from build123d import *

# Parameters (mm, degrees)
BOSS_EXTRUDE1_DEPTH = 3
SKETCH3_W           = 24
SKETCH3_H           = 4
BOSS_EXTRUDE2_DEPTH = 4
SKETCH6_W           = 24
SKETCH6_H           = 4
BOSS_EXTRUDE4_DEPTH = 3
CUT_EXTRUDE1_DEPTH  = 2.3
SKETCH9_W           = 2
SKETCH9_H           = 7
SKETCH9_W_2         = 1.5
BOSS_EXTRUDE5_DEPTH = 3
SKETCH11_W          = 2
SKETCH11_H          = 7
SKETCH11_W_2        = 1.497470588
BOSS_EXTRUDE6_DEPTH = 4
SKETCH10_R          = 1.25
CUT_EXTRUDE2_DEPTH  = 10.5
BOSS_EXTRUDE7_DEPTH = 2


with BuildPart() as part:
    # Sketch1 → Boss-Extrude1 (new body)
    with BuildSketch(Plane(origin=(0, 0, 0), x_dir=(1, 0, 0), z_dir=(0, 1, 0))):
        with BuildLine():
            ThreePointArc((-17.3, 2), (-18.5, 3.2), (-19.7, 2))
            Line((-19.7, 2), (-17.3, 2))
        make_face()
        with BuildLine():
            Line((-17.3, 2), (-19.7, 2))
            ThreePointArc((-19.7, 2), (-18.5, 0.8), (-17.3, 2))
        make_face()
        with BuildLine():
            Line((-23, 2.8), (-23, 2))
            Line((-23, 2), (-23, 1.2))
            ThreePointArc((-23, 1.2), (-22.434314575, 1.434314575), (-22.2, 2))
            ThreePointArc((-22.2, 2), (-22.434314575, 2.565685425), (-23, 2.8))
        make_face()
        with BuildLine():
            Line((-23, 1.2), (-23, 2))
            Line((-23, 2), (-23.8, 2))
            ThreePointArc((-23.8, 2), (-23.565685425, 1.434314575), (-23, 1.2))
        make_face()
        with BuildLine():
            Line((-23.8, 2), (-23, 2))
            Line((-23, 2), (-23, 2.8))
            ThreePointArc((-23, 2.8), (-23.565685425, 2.565685425), (-23.8, 2))
        make_face()
        with BuildLine():
            ThreePointArc((-13.2, 2), (-14, 2.8), (-14.8, 2))
            Line((-14.8, 2), (-13.2, 2))
        make_face()
        with BuildLine():
            Line((-13.2, 2), (-14.8, 2))
            ThreePointArc((-14.8, 2), (-14, 1.2), (-13.2, 2))
        make_face()
        with BuildLine():
            ThreePointArc((-3.2, 2), (-4, 2.8), (-4.8, 2))
            Line((-4.8, 2), (-3.2, 2))
        make_face()
        with BuildLine():
            Line((-3.2, 2), (-4.8, 2))
            ThreePointArc((-4.8, 2), (-4, 1.2), (-3.2, 2))
        make_face()
    extrude(amount=-BOSS_EXTRUDE1_DEPTH)

    # Sketch3 → Boss-Extrude2 (add)
    with BuildSketch(Plane(origin=(0, 0, 0), x_dir=(1, 0, 0), z_dir=(0, 1, 0))):
        with Locations((-13, 2)):
            Rectangle(SKETCH3_W, SKETCH3_H)
    extrude(amount=BOSS_EXTRUDE2_DEPTH)

    # Sketch6 → Boss-Extrude4 (add)
    with BuildSketch(Plane.XY):
        with Locations((-13, 2)):
            Rectangle(SKETCH6_W, SKETCH6_H)
    extrude(amount=BOSS_EXTRUDE4_DEPTH)

    # Sketch7 → Cut-Extrude1 (cut)
    with BuildSketch(Plane(origin=(0, 4, 0), x_dir=(1, 0, 0), z_dir=(0, 1, 0))):
        Polygon((-23, 0.5), (-23, -3), (-17, -3), (-17, 4), (-23, 4), align=None)
    extrude(amount=-CUT_EXTRUDE1_DEPTH, mode=Mode.SUBTRACT)

    # Sketch9 → Boss-Extrude5 (add)
    with BuildSketch(Plane(origin=(0, 4, 0), x_dir=(1, 0, 0), z_dir=(0, 1, 0))):
        with Locations((-24, 0.5)):
            Rectangle(SKETCH9_W, SKETCH9_H)
        with Locations((-16.25, 0.5)):
            Rectangle(SKETCH9_W_2, SKETCH9_H)
    extrude(amount=BOSS_EXTRUDE5_DEPTH)

    # Sketch11 → Boss-Extrude6 (add)
    with BuildSketch(Plane.XY.offset(3)):
        with Locations((-24, 3.5)):
            Rectangle(SKETCH11_W, SKETCH11_H)
        with Locations((-16.251264706, 3.5)):
            Rectangle(SKETCH11_W_2, SKETCH11_H)
    extrude(amount=BOSS_EXTRUDE6_DEPTH)

    # Sketch10 → Cut-Extrude2 (cut, through all)
    with BuildSketch(Plane(origin=(-15.5, 0, 0), x_dir=(0, 0, -1), z_dir=(1, 0, 0))):
        with Locations((1, 5.25)):
            Circle(SKETCH10_R)
        with Locations((-5, 5.25)):
            Circle(SKETCH10_R)
    extrude(amount=-CUT_EXTRUDE2_DEPTH, mode=Mode.SUBTRACT)

    # Sketch12 → Boss-Extrude7 (add)
    with BuildSketch(Plane(origin=(0, 0, -4), x_dir=(-1, 0, 0), z_dir=(0, 0, -1))):
        Polygon((1, 0), (17, 0), (17, 1.7), (17, 1.704314434), (1, 1.704314434), align=None)
        Polygon((23, 0), (25, 0), (25, 1.704314434), (23, 1.704314434), (23, 1.7), align=None)
    extrude(amount=BOSS_EXTRUDE7_DEPTH)


solid = part.part
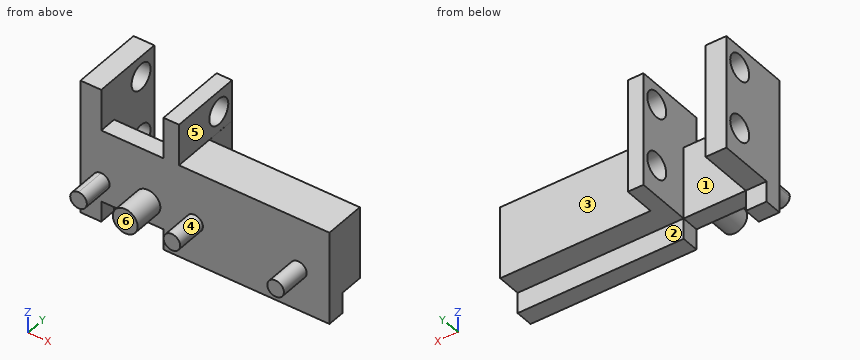
CAD build for the part. Positions are in the model's coordinates, mm. Face numbers are marked on the shaded views. A direction names the side the tool comes from. Round coordinates to 2 decimals unless told otherwise and drop trailing zeros. Loops run counter-clockwise (first coordinate to the right, second up) from the corner with the lowest first, then second, coordinate; pieces in that order, holes last.
(1) Drop flat-ended pins along their axis: pin 1 (1.6 mm diameter, centred on x = -23.5, z = -5, fed in from +Y); pin 2 (1.2 mm diameter, centred on y = 3.5, z = 5, fed in from +X); pin 3 (0.6 mm diameter, centred on x = -24, y = 4, fed in from -Z). Give the stop position or say it passes through.
(2) Two-plate mould, pull along X, no slides. Class the marked faces 4, 5 and 6: +X half, -X half, draft (parallel to the pull), parting line (faces both ways), or undercut.
(3) Which spindle directions (+Z, -Z, +X, -X, +Y, -Y) get a long thin tool onto all of the face, cutting with end or side? Do the marked faces 1, 2 and 3. Say none if no direction does.
(4) Cut at D-D (y = -0.75). Give the cut face in (x, z), plus the area to 3 significant figures.
(5) Cut at C-C (z = 5). Give the cut face in (x, y).
(6) Cut at B-B (x = -16). Give the cut face in (y, z), plus the area to 3 significant figures.
(7) Wall check: line 1 along X through (y, z) = (6, 6.25); line 2 along X through (y, z) = (0.5, -4.25); line 3 along Z through (x, y) = (-3.5, 3.75). Give the ranges that are in metal, low to high.
Findings below:
1. pin 1: stops at y = 1.7
1. pin 2: stops at x = -15.5
1. pin 3: stops at z = -4
2. face 4: undercut
2. face 5: +X half
2. face 6: draft
3. face 1: +Z, -Z, +Y
3. face 2: -Z, +X, -X, +Y
3. face 3: +Z, -Z, +X, +Y
4. outline: circle Ø1.6 at (-23, -2); circle Ø2.4 at (-18.5, -2); circle Ø1.6 at (-14, -2); circle Ø1.6 at (-4, -2)
4. area: 10.6 mm2
5. outline: (-25, 0) - (-23, 0) - (-23, 4) - (-25, 4) - close; (-25, 6.5) - (-23, 6.5) - (-23, 7) - (-25, 7) - close; (-17, 0) - (-15.5, 0) - (-15.5, 4) - (-17, 4) - close; (-17, 6.5) - (-15.5, 6.5) - (-15.5, 7) - (-17, 7) - close
6. outline: (0, -6) - (1.7, -6) - (1.7, -4) - (7, -4) - (7, 7) - (0, 7) - close; hole circle Ø2.5 at (5.25, -1); hole circle Ø2.5 at (5.25, 5)
6. area: 70.6 mm2
7. line 1: x = -25 to -23, -17 to -15.5
7. line 2: x = -25 to -23, -17 to -1
7. line 3: z = -4 to 3
